Here's how the part is built. I have some questions about the finished solid (model axes, mm). Face numbers are marked on the shaded views. A direction names the side the tool comes from. Coordinates: 2 decimals unless noted, no trailing zeros. Loops run counter-clockwise (first coordinate to the right, second up) from the corner with the lowest first, then second, coordinate; pieces in that order, holes last. Notation, with made-up numbers: (56.5, -36) - (115.5, -36) arc R26 cw to (115.5, -4) - close; hole circle Ø1 at (55.25, -2.5). An arc over 180 degrees is marked (long way). Use a Markdown table: item, result.
Autodesk Inventor part; units mm, degrees
ref_plane "YZ Plane" through (0, 0, 0) normal (1, 0, 0) x (0, 1, 0)
ref_plane "XZ Plane" through (0, 0, 0) normal (0, 1, 0) x (-1, 0, 0)
ref_plane "XY Plane" through (0, 0, 0) normal (0, 0, 1) x (1, 0, 0)
sketch "Sketch1" plane through (0, 0, 0) normal (0, 0, 1) x (1, 0, 0)
  circle A0 centre (0, 0) radius 35
  point P0 (0, 35)
  point P1 (0, -35)
  dimension "d0" = 70
extrude "Extrusion1" add sketch "Sketch1" along normal blind 8
sketch "Sketch3" plane through (0, 0, 8) normal (0, 0, 1) x (1, 0, 0)
  circle A0 centre (0, 0) radius 57.5
  dimension "d8" = 115
extrude "Extrusion3" add sketch "Sketch3" along normal blind 8
sketch "Sketch7" plane through (0, 0, 16) normal (0, 0, 1) x (1, 0, 0)
  line L0 (-15, 25.9808) -> (0, 0)
  line L1 (0, 80.5) -> (0, -80.5)
  dimension "d25" = 30
  dimension "d26" = 30
hole "Hole2" at (-15, 25.9808, 16) direction (0, 0, -1) diameter 3.4 end through all counterbore diameter 7 counterbore depth 4
pattern_circular "Circular Pattern1" count 6 over 360 about axis through (0, 0, -10) along (0, 0, 1) of "Hole2"
sketch "Sketch12" plane through (0, 0, 16) normal (0, 0, 1) x (1, 0, 0)
  line L0 (-12.4233, 46.3644) -> (0, 0)
  line L1 (0, 80.5) -> (0, -80.5)
  dimension "d77" = 15
  dimension "d78" = 48
hole "Hole6" at (-12.4233, 46.3644, 16) direction (0, 0, -1) diameter 2.459 end through all
pattern_circular "Circular Pattern2" count 12 over 360 about axis through (0, 0, -10) along (0, 0, 1) of "Hole6"
sketch "Sketch8" plane through (0, 0, 16) normal (0, 0, 1) x (1, 0, 0)
  line L0 (0, 23.094) -> (20, 11.547)
  line L1 (20, 11.547) -> (20, -11.547)
  line L2 (20, -11.547) -> (0, -23.094)
  line L3 (0, -23.094) -> (-20, -11.547)
  line L4 (-20, -11.547) -> (-20, 11.547)
  line L5 (-20, 11.547) -> (0, 23.094)
  point P0 (0, 0)
  point P1 (0, 0)
  dimension "d37" = 40
extrude "Extrusion4" cut sketch "Sketch8" against normal through all
properties part number "201-"
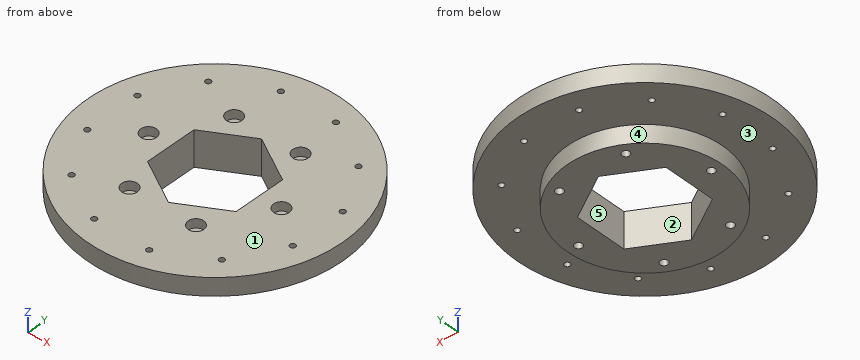
Q1. Please list where these lines run through material, in increasing order: L1, parallel to Y at x = 47, z = 13.75; L2, parallel to Y at x = 13, z = 14.5; L3, parallel to Y at x = -14, z = 3.75. Write a range as from..to.
Check values:
| item | result |
|---|---|
| L1 | -33.12..-13.48, -11.37..11.37, 13.48..33.12 |
| L2 | -56.01..-47.45, -45.28..-28.85, -23.11..-15.59, 15.59..23.11, 28.85..45.28, 47.45..56.01 |
| L3 | -32.08..-27.36, -24.61..-15.01, 15.01..24.61, 27.36..32.08 |
Q2. Which directions (+Z, -Z, +X, -X, +Y, -Y) give clear straight access to the entire face, cutting with the end or side of a thin tool? Please do the marked faces 1 and 2.
Check values:
| item | result |
|---|---|
| face 1 | +Z, +X, -X, +Y, -Y |
| face 2 | +Z, -Z |
Q3. If we mould it in two halves opening along Y, with no side actions, what happens to the marked faces 3, 4 and 5? For each: pulls with the +Y half, pulls with the -Y half, needs draft (parallel to the pull), parting line crosses it, or undercut.
Check values:
| item | result |
|---|---|
| face 3 | needs draft |
| face 4 | parting line crosses it |
| face 5 | undercut |
Q4. I want a section at C-C, the plane z = 1.5. Write out the boundary of the cut face in (x, y), then the cut area to 3 significant figures.
Check values:
| item | result |
|---|---|
| outline | circle Ø70 at (0, 0); hole circle Ø3.4 at (-30, 0); hole (-20, -11.55) - (0, -23.09) - (20, -11.55) - (20, 11.55) - (0, 23.09) - (-20, 11.55) - close; hole circle Ø3.4 at (-15, -25.98); hole circle Ø3.4 at (-15, 25.98); hole circle Ø3.4 at (15, -25.98); hole circle Ø3.4 at (15, 25.98); hole circle Ø3.4 at (30, 0) |
| area | 2,410 mm^2 |
Q5. I want a section at B-B, the plane y = 9. Write out the boundary of the cut face in (x, z), then the cut area to 3 significant figures.
Check values:
| item | result |
|---|---|
| outline | (-56.79, 8) - (-33.82, 8) - (-33.82, 0) - (-20, 0) - (-20, 16) - (-56.79, 16) - close; (20, 0) - (33.82, 0) - (33.82, 8) - (56.79, 8) - (56.79, 16) - (20, 16) - close |
| area | 810 mm^2 |
Q6. I want a section at D-D, the plane y = 43. Write out the boundary of the cut face in (x, z), then the cut area to 3 significant figures.
Check values:
| item | result |
|---|---|
| outline | (-38.17, 8) - (38.17, 8) - (38.17, 16) - (-38.17, 16) - close |
| area | 611 mm^2 |
Q7. Will these pins go through, and if not, where does the flat tip stop? P1, Ø5.5, axis at x = -14.5, y = -24.5, coming from the +Z side; P2, Ø2, axis at x = -15, z = 6, coming from the -Y side; P3, Ø4, axis at x = -46.36, y = 12.42, coming from the -Z side; P4, Ø4, axis at x = 15, y = -25.98, coming from the +Z side.
Check values:
| item | result |
|---|---|
| P1 | z = 16 |
| P2 | y = -32.08 |
| P3 | z = 8 |
| P4 | z = 12 |
Q8. I want a section at A-A, the plane x = 15. Write out the boundary of the cut face in (y, z), then the cut area to 3 significant figures.
Check values:
| item | result |
|---|---|
| outline | (-55.51, 8) - (-31.62, 8) - (-31.62, 0) - (-27.68, 0) - (-27.68, 12) - (-29.48, 12) - (-29.48, 16) - (-55.51, 16) - close; (-24.28, 0) - (-14.43, 0) - (-14.43, 16) - (-22.48, 16) - (-22.48, 12) - (-24.28, 12) - close; (14.43, 0) - (24.28, 0) - (24.28, 12) - (22.48, 12) - (22.48, 16) - (14.43, 16) - close; (27.68, 0) - (31.62, 0) - (31.62, 8) - (55.51, 8) - (55.51, 16) - (29.48, 16) - (29.48, 12) - (27.68, 12) - close |
| area | 795 mm^2 |
